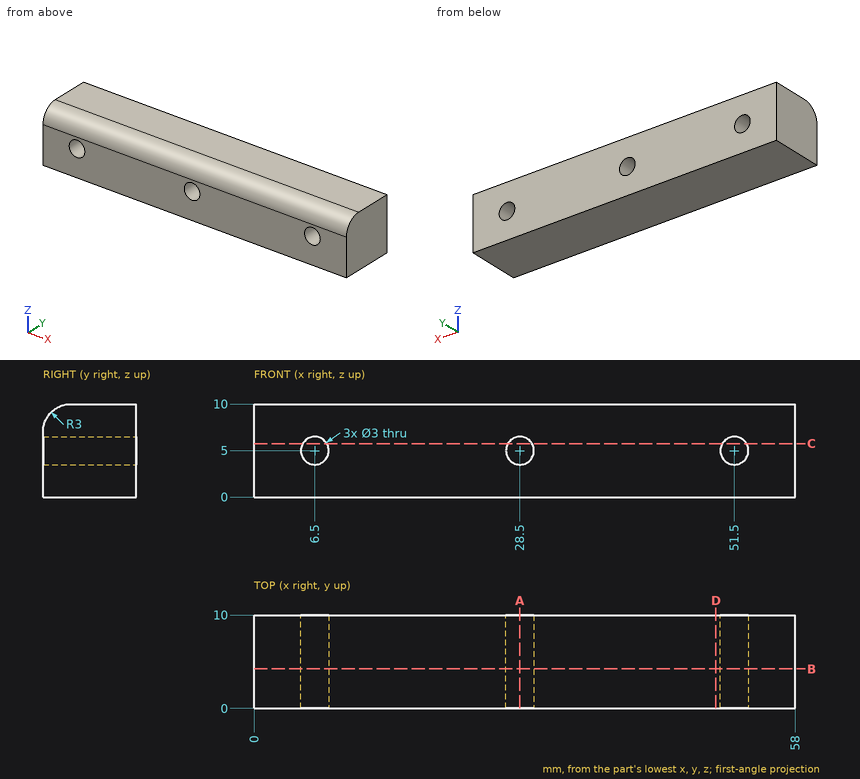
The figure shows three views and two pictorial views of one solid part (mm, origin at its lowest corner). Answer the questions. Coordinates: 2 decimals unless noted, no trailing zeros. Loops run counter-clockwise (first coordinate to the right, second up) from the corner with the lowest first, then second, coordinate; pieces in that order, holes last.
(1) The part is cut by section D-D (x = 49.5). Determine the outline of the cut face in (y, z).
Solution:
outline: (0, 0) - (10, 0) - (10, 10) - (3, 10) arc R3 ccw to (0, 7) - close
(2) The part is cut by section C-C (z = 5.75). Determine the outline of the cut face in (x, y).
Solution:
outline: (0, 0) - (5.2, 0) - (5.2, 10) - (0, 10) - close; (7.8, 0) - (27.2, 0) - (27.2, 10) - (7.8, 10) - close; (29.8, 0) - (50.2, 0) - (50.2, 10) - (29.8, 10) - close; (52.8, 0) - (58, 0) - (58, 10) - (52.8, 10) - close
(3) A flat-ended cylindrical pin translates along its axis: pin 1 Ø2.5 at (x, z) = (51.5, 5) entering from +Y. Find the tip coordinate at first contact, or state that the pin passes through.
Solution:
pin 1: passes through
(4) The part is cut by section A-A (x = 28.5). Determine the outline of the cut face in (y, z), and give its area (3 significant figures).
Solution:
outline: (0, 0) - (10, 0) - (10, 3.5) - (0, 3.5) - close; (0, 6.5) - (10, 6.5) - (10, 10) - (3, 10) arc R3 ccw to (0, 7) - close
area: 68.1 mm2
(5) The part is cut by section B-B (y = 4.25). Determine the outline of the cut face in (x, z), and give its area (3 significant figures).
Solution:
outline: (0, 0) - (58, 0) - (58, 10) - (0, 10) - close; hole circle Ø3 at (6.5, 5); hole circle Ø3 at (28.5, 5); hole circle Ø3 at (51.5, 5)
area: 559 mm2
(6) Consider line 1 along Z through (x, y) = (51.5, 7.5); line 2 along X through (y, z) = (9.5, 4); line 3 along X through (y, z) = (7.75, 4.25). Determine where each line is inside the solid, lowest interval first.
Solution:
line 1: z = 0 to 3.5, 6.5 to 10
line 2: x = 0 to 5.38, 7.62 to 27.38, 29.62 to 50.38, 52.62 to 58
line 3: x = 0 to 5.2, 7.8 to 27.2, 29.8 to 50.2, 52.8 to 58
